```python
from build123d import *

# Parameters (mm, degrees)
BOSS_EXTRUDE1_DEPTH = 3
FILLET1_R           = 5
FILLET2_R           = 2.5


with BuildPart() as part:
    # Sketch1 → Boss-Extrude1 (new body)
    with BuildSketch(Plane.XY):
        Polygon((-5, -25), (-5, -159), (-25, -159), (-25, -169), (-16.1, -169), (-16.1, -166.5), (-18.6, -166.5), (-18.6, -164.5), (-16.1, -164.5), (-16.1, -162), (-13.9, -162), (-13.9, -164.5), (-11.4, -164.5), (-11.4, -166.5), (-13.9, -166.5), (-13.9, -169), (-5, -169), (-5, -175), (-1.5, -175), (-1.5, -159), (1.5, -159), (1.5, -175), (5, -175), (5, -169), (13.9, -169), (13.9, -166.5), (11.4, -166.5), (11.4, -164.5), (13.9, -164.5), (13.9, -162), (16.1, -162), (16.1, -164.5), (18.6, -164.5), (18.6, -166.5), (16.1, -166.5), (16.1, -169), (25, -169), (25, -159), (5, -159), (5, -25), (28.8675, -25), (0, 25), (-28.8675, -25), align=None)
    extrude(amount=BOSS_EXTRUDE1_DEPTH)

    # Fillet1
    fillet1_edges = [part.edges().sort_by_distance(p)[0] for p in [
        (5, -25, 1.5),
        (5, -159, 1.5),
        (25, -159, 1.5),
        (-25, -159, 1.5),
        (-5, -159, 1.5),
        (-5, -25, 1.5),
    ]]
    fillet(fillet1_edges, radius=FILLET1_R)

    # Fillet2
    fillet2_edges = [part.edges().sort_by_distance(p)[0] for p in [
        (0, 25, 1.5),
        (28.8675, -25, 1.5),
        (-28.8675, -25, 1.5),
    ]]
    fillet(fillet2_edges, radius=FILLET2_R)


solid = part.part
```
CAD build for the part. Positions are in the model's coordinates, mm. A direction names the side the tool comes from. Coordinates: 2 decimals unless noted, no trailing zeros. Loops run counter-clockwise (first coordinate to the right, second up) from the corner with the lowest first, then second, coordinate; pieces in that order, holes last. Notation, with made-up numbers: (86, -12.75) - (135, -12.75) arc R23 ccw to (135, 4.25) - close; hole circle Ø4 at (20, -15). An arc over 180 degrees is marked (long way). Return JSON: item names as keys, results as strings.
1. Drop flat-ended pins along their axis: pin 1 (5 mm diameter, centred on x = 20, y = -28.5, fed in from +Z); pin 2 (1.6 mm diameter, centred on y = -165, z = 1, fed in from +X); pin 3 (1.5 mm diameter, centred on y = -87, z = 2, fed in from -X); pin 4 (1.5 mm diameter, centred on y = -4.5, z = 0.5, fed in from +X). Give the stop position or say it passes through.
Result:
{"pin 1": "passes through", "pin 2": "stops at x = 25", "pin 3": "stops at x = -5", "pin 4": "stops at x = 17.46"}
2. Band-saw the part on B-B (y = -19.5). Give the cut face in (x, z), and give its area (3 significant figures).
Result:
{"outline": "(-25.69, 0) - (25.69, 0) - (25.69, 3) - (-25.69, 3) - close", "area": "154 mm2"}
3. Band-saw the part on A-A (y = -150). Give the cut face in (x, z).
Result:
{"outline": "(-5, 0) - (5, 0) - (5, 3) - (-5, 3) - close"}
4. Probe L1, parallel to X at y = -133, z = 2.3; L2, parallel to Y at x = -7.5, z = 1.6; L3, parallel to Y at x = -14.5, z = 0.1. List the from-to ranges inside material, lowest first. Write a range as from..to.
Result:
{"L1": "x = -5..5", "L2": "y = -169..-158.33, -25.67..12.01", "L3": "y = -162..-159, -25..-0.11"}
5. 3-axis set-ups, long thin cutter, end or side, ignore diameter. For faces 1 (the flat face through (-14.26, 0.3, 1.48)), 2 (the cylindrical face through (24, -161, 2)), 3 (the cylindrical face through (-23, -160, 2)): which of +Z, -Z, +X, -X, +Y, -Y reach the whole face in a straight line?
Result:
{"face 1": "+Z, -Z, -X, +Y", "face 2": "+Z, -Z, +X", "face 3": "+Z, -Z, -X"}
6. Mould opens along Y. For faces 4 (the flat face through (14.606, -0.298, 1.479)), 5 (the cylindrical face through (-6, -157, 2)), 6 (the flat face through (4, -61, 0)) say: released by +Y, released by -Y, zero draft, split by the parting line, or undercut.
Result:
{"face 4": "released by +Y", "face 5": "undercut", "face 6": "zero draft"}
